Autodesk Fusion 360 part; units mm, degrees
sketch "Boceto1" plane through (0, 0, 0) normal (0, 1, 0) x (1, 0, 0)
  circle A0 centre (0, 0) radius 3
  dimension "d1" = 6
sketch "Boceto3" plane through (0, 0, 0) normal (0, -1, 0) x (1, 0, 0)
  circle A0 centre (0, 0) radius 3
  circle A1 centre (0, 0) radius 1.525
  dimension "d8" = 3.05
extrude "Extruir2" add sketch "Boceto1" along normal blind 50
sketch "Boceto4" plane through (0, 50, 0) normal (0, 1, 0) x (-1, 0, 0)
  circle A0 centre (0, 0) radius 3
  circle A1 centre (0, 0) radius 1.525
  dimension "d14" = 3.05
hole "Agujero3" at (0, 50, 0) direction (0, -1, 0) diameter 3 depth 15 tip angle 118
hole "Agujero4" at (0, 0, 0) direction (0, 1, 0) diameter 3 depth 15 tip angle 118
Input: part model. Units: mm. Frame: model coordinates. A direction names the side the tool comes from. Give positions to 0.01 mm unless a question says otherwise; leave off trailing zeros. Loops run counter-clockwise (first coordinate to the right, second up) from the corner with the lowest first, then second, coordinate; pieces in that order, holes last. Notation, with made-up numbers: M 82,17 L 117,17 A21 cw 117,41 Z; hole C -22.5,-12.5 d6. An arc over 180 degrees is marked long. Use CSV: the item, a comma, the result in double quotes.
(1) Pin query (flat end, axial travel): P1, Ø1.5, axis at x = 0.5, z = 2, coming from the -Y side; P2, Ø1.8, axis at x = 0, z = 0, coming from the +Y side; P3, Ø1, axis at x = -2, y = 15.5, coming from the +Z side; P4, Ø2, axis at x = 1.5, y = 43, coming from the -Z side. Return the tip coordinate at first contact, or that it passes through.
Outcome:
P1,"stops at y = 0"
P2,"stops at y = 34.64"
P3,"stops at z = 2.6"
P4,"stops at z = -2.96"
(2) Material intervals for L1, parallel to X at y = 11.75, z = 0; L2, parallel to Z at x = -2.6, y = 11, sorted ascending. Write a range as [from, to].
Outcome:
L1,"x = [-3, -1.5], [1.5, 3]"
L2,"z = [-1.5, 1.5]"
(3) Section B-B, the plane y = 24. Return loops of the section in (x, z).
Outcome:
outline,"C 0,0 d6"
(4) Section C-C, the plane z = -1.95. Return loops of the section in (x, y).
Outcome:
outline,"M -2.28,0 L 2.28,0 L 2.28,50 L -2.28,50 Z"
(5) Section D-D, the plane x = -2.35. Return loops of the section in (y, z), plus the area to 3 significant figures.
Outcome:
outline,"M 0,-1.86 L 50,-1.86 L 50,1.86 L 0,1.86 Z"
area,"186 mm²"
(6) Set-up query: faces 1 (the face through (1.3, 0, 1.3)), 2 (the face through (-0.07, 7.6, 1.5)). Return all of +Z, -Z, +X, -X, +Y, -Y with unobstructed straight access to the full face (end or side cutting, diameter ignored); none if empty.
Outcome:
face 1,"+Z, -Z, +X, -X, -Y"
face 2,"-Y"
(7) Section A-A, the plane y = 37.5. Return loops of the section in (x, z), plus the area to 3 significant figures.
Outcome:
outline,"C 0,0 d6; hole C 0,0 d3"
area,"21.2 mm²"
(8) Pull-direction query (Z, two-part tool) for faces 3 (the face through (-0.07, 42.4, -1.5)), 4 (the face through (1.3, 50, 1.3)), 5 (the face through (0.078, 15.745, -0.248)), 6 (the face through (-3, 25, 0)); classes: pulls with the +Z half, pulls with the -Z half, needs draft (parallel to the pull), parting line crosses it, or undercut.
Outcome:
face 3,"undercut"
face 4,"needs draft"
face 5,"undercut"
face 6,"parting line crosses it"
